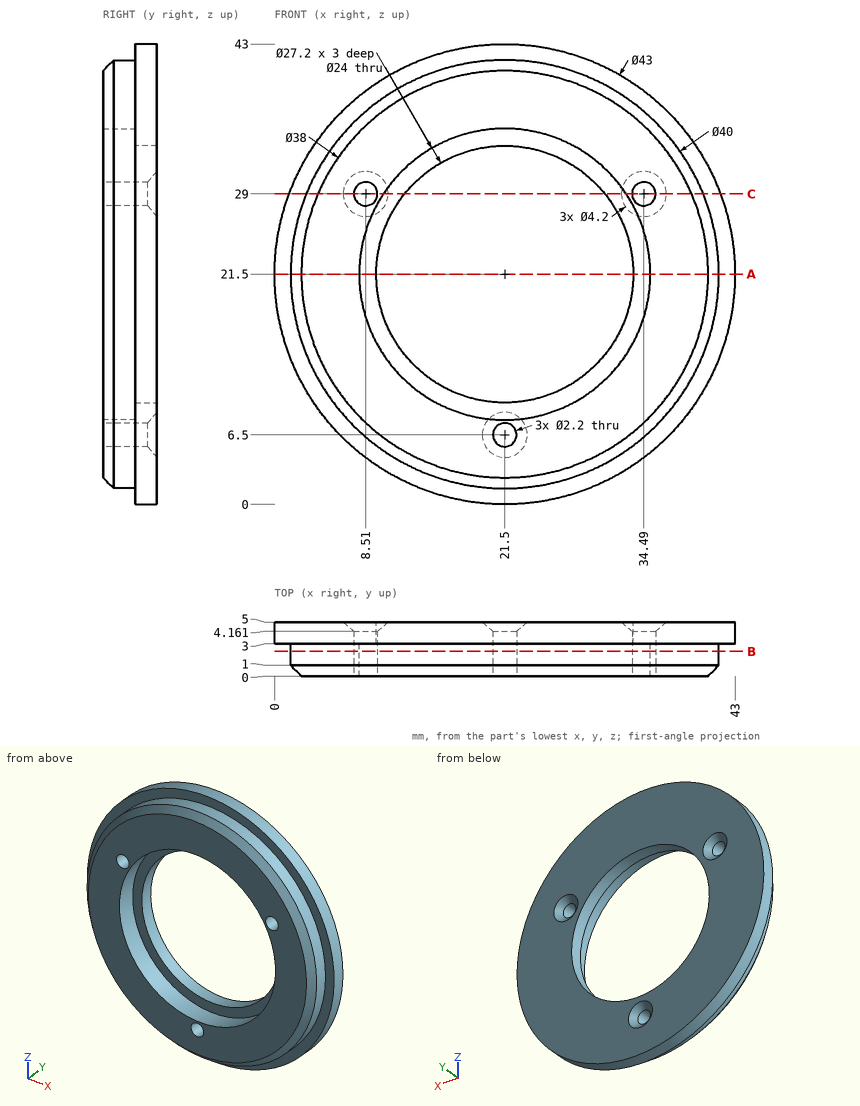
Job drawing, mm, ordinate dimensions from the low corner. One solid piece. Give positions to 0.01 mm unless a question says otherwise; leave off trailing zeros. Loops run counter-clockwise (first coordinate to the right, second up) from the corner with the lowest first, then second, coordinate; pieces in that order, holes last. Notation, with made-up numbers: M 66,-3.5 L 107,-3.5 A26 cw 107,10.5 Z; hole C -13,50 d6. An arc over 180 degrees is marked long. Return JSON: item names as keys, results as strings.
1) Saw through at A-A, the plane z = 21.5. List the corners of the cut face in (x, y), then the cut area to 3 significant figures.
Calculated:
{"outline": "M 0,3 L 1.5,3 L 1.5,1 L 2.5,0 L 7.9,0 L 7.9,3 L 9.5,3 L 9.5,5 L 0,5 Z; M 33.5,3 L 35.1,3 L 35.1,0 L 40.5,0 L 41.5,1 L 41.5,3 L 43,3 L 43,5 L 33.5,5 Z", "area": "75.4 mm2"}
2) Saw through at C-C, the plane z = 29. Count the separate pieces of the cut face and the enclosed holes in it.
Calculated:
{"separate pieces": "4", "enclosed holes": "0"}
3) Saw through at B-B, the plane y = 2.3. List the corners of the cut face in (x, z).
Calculated:
{"outline": "C 21.5,21.5 d40; hole C 8.51,29 d2.2; hole C 21.5,21.5 d27.2; hole C 21.5,6.5 d2.2; hole C 34.49,29 d2.2"}
4) Flat gauge pins, fed straight in: pin 1 Ø2.5 at (x, z) = (34.49, 29) entering from +Y; pin 2 Ø21.5 at (x, z) = (21.5, 21.5) entering from -Y; pin 3 Ø3 at (x, z) = (8.51, 29) entering from +Y; pin 4 Ø1.5 at (x, y) = (34, 0.5) entering from -Z (1 decimal). Where does each tip first touch, or does it go through?
Calculated:
{"pin 1": "stops at y = 4.29", "pin 2": "passes through", "pin 3": "stops at y = 4.5", "pin 4": "stops at z = 5.5"}
5) Drill centre lines: line 1 (X direction, y = 4, z = 21.5); line 2 (X direction, y = 1.3, z = 21.5); line 3 (X direction, y = 1.5, z = 29) (1 decimal). Where is each one in solid material? Low to high.
Calculated:
{"line 1": "x = 0 to 9.5, 33.5 to 43", "line 2": "x = 1.5 to 7.9, 35.1 to 41.5", "line 3": "x = 3 to 7.4, 9.6 to 10.2, 32.8 to 33.4, 35.6 to 40"}
